Check sheet for the modelled part. Datum: model origin and axes. Units: mm. Coordinates: 2 decimals unless noted, no trailing zeros. Loops run counter-clockwise (first coordinate to the right, second up) from the corner with the lowest first, then second, coordinate; pieces in that order, holes last. Notation, with made-up numbers: M 72.25,-6.5 L 97.25,-6.5 A18 cw 97.25,6.5 Z; hole C 15.5,63 d8. An arc over 180 degrees is marked long. Use CSV: the item, a comma, the result in double quotes. Start each with the question number.
(1) Section check B-B on y = 17.5. Record the cut outline in (x, z).
(2) Section check C-C on x = 2. Record the cut outline in (y, z), and give its area (3 significant figures).
(3) Section check D-D on z = -9. Give the number of separate pieces and of enclosed holes in the cut face, and give its area (3 significant figures).
(4) Scan lines: line 1 (Y direction, x = -41, z = -10.5); line 2 (Y direction, x = -16, z = 11.7); line 3 (X direction, y = -14, z = -16). Record each from-to range of solid material in increasing order.
(5) Go/stop test with flat-tipped pins: pin 1 Ø2.5 at (x, y) = (-41, 65) entering from -Z; pin 2 Ø4 at (x, y) = (6, 26) entering from -Z; pin 3 Ø16 at (x, y) = (-17, 13.5) entering from -Z. Record where each tip stops, or that it passes through.
(6) Draft check along X on faces 1 (the flat face through (-44, 25, -2)), 2 (the flat face through (-38, 64, -7)). Enter one of: pulls with the +X half, pulls with the -X half, needs draft (parallel to the pull), parting line crosses it, or undercut.
(7) Section check A-A on x = -16. Record the cut outline in (y, z).
Autodesk Inventor part; units mm, degrees
ref_plane "YZ Plane" through (0, 0, 0) normal (1, 0, 0) x (0, 1, 0)
ref_plane "XZ Plane" through (0, 0, 0) normal (0, 1, 0) x (-1, 0, 0)
ref_plane "XY Plane" through (0, 0, 0) normal (0, 0, 1) x (1, 0, 0)
sketch "Skizze1" plane through (0, 0, 0) normal (1, 0, 0) x (0, 1, 0)
  circle A0 centre (0, 0) radius 7.75
  line L0 (0, 0) -> (7.75, 0) construction
  circle A1 centre (17, 0) radius 7.75
  circle A2 centre (34, 0) radius 7.75
  circle A3 centre (51, 0) radius 7.75
  line L1 (66, 3.75) -> (-15, 3.75)
  line L2 (-15, 3.75) -> (-15, 9.75)
  line L3 (-15, 9.75) -> (66, 9.75)
  line L4 (66, 9.75) -> (66, 3.75)
  point P0 (24.75, 0)
  point P1 (41.75, 0)
  point P2 (58.75, 0)
  point P3 (66, 6.75)
  point P4 (-6.7823, 3.75)
  point P5 (6.7823, 3.75)
  point P6 (10.2177, 3.75)
  point P7 (23.7823, 3.75)
  point P8 (27.2177, 3.75)
  point P9 (40.7823, 3.75)
  point P10 (44.2177, 3.75)
  point P11 (57.7823, 3.75)
  dimension "d0" = 15.5
  dimension "d3" = 17
  dimension "a" = 9.75
  dimension "b" = 15
  dimension "d10" = 15
  dimension "d11" = 6
extrude "Extrusion1" add sketch "Skizze1" along normal blind 10 contours A0 L1 L2 L3 L4 A3 A2 A1
sketch "Skizze2" plane through (0, -15, 9.75) normal (0, 0, 1) x (1, 0, 0)
  line L0 (0, 81) -> (10, 81)
  line L1 (10, 81) -> (-16, 81)
  line L2 (-16, 81) -> (-16, 0)
  line L3 (-16, 0) -> (10, 0)
  line L4 (10, 0) -> (10, 81)
  line L5 (0, 0) -> (10, 0)
  point P0 (0, 15)
  dimension "d14" = 26
extrude "Extrusion2" add sketch "Skizze2" along normal blind 3
sketch "Skizze3" plane through (10, 0, 0) normal (1, 0, 0) x (0, 0, -1)
  line L0 (-12.75, 66) -> (-12.75, -15)
  line L1 (-12.75, 66) -> (17, 66)
  line L2 (17, 66) -> (17, -15)
  line L3 (17, -15) -> (-12.75, -15)
  line L4 (-12.75, -15) -> (-12.75, 66)
  line L5 (-3.75, -15) -> (-12.75, -15) construction
  circle A0 centre (17, 51) radius 2.5 construction
  point P0 (0, 0)
  point P1 (-12.75, -15)
extrude "Extrusion3" add sketch "Skizze3" along normal blind 2
sketch "Skizze4" plane through (-16, -15, 9.75) normal (0, -1, 0) x (1, 0, 0)
  line L0 (0, 3) -> (28, 3)
  line L1 (28, -26.75) -> (28, 3)
  line L2 (0, 3) -> (28, 3)
  line L3 (28, 3) -> (28, -26.75)
  line L4 (28, -26.75) -> (0, -26.75)
  line L5 (0, -26.75) -> (0, 3)
  point P0 (16, -9.75)
extrude "Extrusion4" add sketch "Skizze4" along normal blind 2
sketch "Skizze5" plane through (-16, 66, 9.75) normal (0, 1, 0) x (1, 0, 0)
  line L0 (0, 0) -> (0, 26.75)
  line L1 (28, -3) -> (0, -3)
  line L2 (0, -3) -> (0, 26.75)
  line L3 (0, 26.75) -> (28, 26.75)
  line L4 (28, 26.75) -> (28, -3)
  point P0 (16, 9.75)
extrude "Extrusion5" add sketch "Skizze5" along normal blind 2
sketch "Skizze6" plane through (10, -15, -17) normal (0, 0, -1) x (-1, 0, 0)
  line L0 (-2, -2) -> (26, -2)
  line L1 (-2, -2) -> (4, -2)
  line L2 (4, -2) -> (4, 4)
  line L3 (4, 4) -> (-2, 4)
  line L4 (-2, 4) -> (-2, -2)
  line L5 (-2, 83) -> (26, 83)
  line L6 (-2, 83) -> (4, 83)
  line L7 (4, 83) -> (4, 77)
  line L8 (4, 77) -> (-2, 77)
  line L9 (-2, 77) -> (-2, 83)
  point P0 (10, 15)
  point P1 (4, 83)
  dimension "d23" = 6
extrude "Extrusion6" add sketch "Skizze6" against normal up to surface (20.75 mm away)
fillet "Rundung1" radius 1 8 edges at (10, -11, -6.625) (6, -11, -6.625) (6, -15, -6.625) (12, -17, -2.125) (12, 68, -2.125) (10, 62, -6.625) (6, 62, -6.625) (6, 66, -6.625)
sketch "Skizze8" plane through (5, 66, -17) normal (0, 0, -1) x (-1, 0, 0)
  arc A0 (-6, 2) -> (-7, 1) centre (-6, 1) ccw construction
  arc A1 (-2, -4) -> (-1, -3) centre (-2, -3) ccw construction
  line L0 (-6, 1) -> (-2, -3) construction
  arc A2 (-7, -82) -> (-6, -83) centre (-6, -82) ccw construction
  line L1 (-6, -82) -> (-2, -78) construction
  point P0 (5, -66)
  point P1 (-4, -80)
  point P2 (-4, -1)
hole "Bohrung1" at (9, -14, -17) at (9, 65, -17) direction (0, 0, 1) diameter 3.2 depth 3
hole "Bohrung2" at (9, 65, -17) at (9, -14, -17) direction (0, 0, 1) diameter 2.4 depth 15
mirror "Spiegeln1" about plane through (-16, 66, 9.75) normal (-1, 0, 0) of "Extrusion1", "Extrusion2", "Extrusion3", "Extrusion4", "Extrusion5", "Extrusion6", "Rundung1", "Bohrung1", "Bohrung2"
sketch "Skizze7" plane through (0, -15, 9.75) normal (0, 0, -1) x (-1, 0, 0)
  line L0 (0, 81) -> (0, 0)
  line L1 (32, 0) -> (0, 0)
  line L2 (32, 81) -> (32, 0)
  line L3 (0, 81) -> (32, 81)
  point P0 (0, 15)
extrude "Extrusion7" add sketch "Skizze7" along normal blind 1
fillet "Rundung2" radius 1 4 edges at (-44, 25.5, 12.75) (-16, -17, 12.75) (12, 25.5, 12.75) (-16, 68, 12.75)
sketch "Skizze9" plane through (0, -15, 8.75) normal (0, 0, -1) x (-1, 0, 0)
  line L0 (0, 81) -> (32, 81) construction
  line L1 (16, 81) -> (16, 32.5) construction
  line L2 (16, 32.5) -> (16, 7.5) construction
  line L3 (16, 7.5) -> (16, 0) construction
  line L4 (32, 0) -> (0, 0) construction
  point P0 (0, 15)
  dimension "d44" = 25
  dimension "d52" = 7.5
hole "Bohrung3" at (-16, 17.5, 8.75) at (-16, -7.5, 8.75) direction (0, 0, 1) diameter 3.4 end through all countersink diameter 7.5 countersink angle 90
properties part number "BatteryCase_Botton"
Outcome:
1,outline,"M -44,-17 L -42,-17 L -42,7.73 L -32,7.73 L -32,8.75 L -19.75,8.75 L -17.7,10.8 L -17.7,12.75 L -43,12.75 A1 ccw -44,11.75 Z; M -14.3,10.8 L -12.25,8.75 L 0,8.75 L 0,7.73 L 10,7.73 L 10,-17 L 12,-17 L 12,11.75 A1 ccw 11,12.75 L -14.3,12.75 Z"
2,outline,"M -17,-17 L -15,-17 L -15,3.75 L -6.78,3.75 A7.75 cw 6.78,3.75 L 10.22,3.75 A7.75 cw 23.78,3.75 L 27.22,3.75 A7.75 cw 40.78,3.75 L 44.22,3.75 A7.75 cw 57.78,3.75 L 66,3.75 L 66,-17 L 68,-17 L 68,11.75 A1 ccw 67,12.75 L -16,12.75 A1 ccw -17,11.75 Z"
2,area,"693 mm²"
3,separate pieces,"1"
3,enclosed holes,"5"
3,area,"594 mm²"
4,line 1,"y = -17 to -15.2, -12.8 to -11, 62 to 63.8, 66.2 to 68"
4,line 2,"y = -17 to -9.2, -5.8 to 15.8, 19.2 to 68"
4,line 3,"x = -44 to -42.6, -39.4 to -38, 6 to 7.4, 10.6 to 12"
5,pin 1,"stops at z = -14"
5,pin 2,"stops at z = 3.75"
5,pin 3,"stops at z = 8.75"
6,face 1,"pulls with the -X half"
6,face 2,"undercut"
7,outline,"M -17,-17 L -15,-17 L -15,8.75 L -11.25,8.75 L -9.2,10.8 L -9.2,12.75 L -16,12.75 A1 ccw -17,11.75 Z; M -5.8,10.8 L -3.75,8.75 L 13.75,8.75 L 15.8,10.8 L 15.8,12.75 L -5.8,12.75 Z; M 19.2,10.8 L 21.25,8.75 L 66,8.75 L 66,-17 L 68,-17 L 68,11.75 A1 ccw 67,12.75 L 19.2,12.75 Z"
